```python
from build123d import *

# Parameters (mm, degrees)
SKETCH1_R           = 38.1
BOSS_EXTRUDE1_DEPTH = 4.826
SKETCH2_R           = 38.1
BOSS_EXTRUDE2_DEPTH = 3.302
BOSS_EXTRUDE2_DRAFT = -70
SKETCH3_R           = 47.172170439
BOSS_EXTRUDE3_DEPTH = 3.81
SKETCH4_R           = 46.472170439
CUT_EXTRUDE1_DEPTH  = 0.2
SKETCH6_R           = 34.772170439
SKETCH6_R_2         = 12.7
CUT_EXTRUDE2_DEPTH  = 2.7
SKETCH8_R           = 12.7
BOSS_EXTRUDE4_DEPTH = 50.8
SKETCH10_R          = 7.35
CUT_EXTRUDE5_DEPTH  = 3
SKETCH13_R          = 6.4
CUT_EXTRUDE9_DEPTH  = 92.577748235
SKETCH15_R          = 37.5
BOSS_EXTRUDE6_DEPTH = 8
CUT_EXTRUDE10_REACH = 99.233
SKETCH16_R          = 2
SKETCH16_R_2        = 5.35
SKETCH17_R          = 20.71
SKETCH17_R_2        = 19.21
CUT_EXTRUDE11_DEPTH = 3
SKETCH19_R          = 4.5
CUT_EXTRUDE12_DEPTH = 3.75


with BuildPart() as part:
    # Sketch1 → Boss-Extrude1 (new body)
    with BuildSketch(Plane(origin=(0, 0, 0), x_dir=(1, 0, 0), z_dir=(0, 1, 0))):
        with Locations(Location((0, 0, 0), (0, 0, 270))):
            Circle(SKETCH1_R)
    extrude(amount=BOSS_EXTRUDE1_DEPTH)


with BuildPart() as boss_extrude2_tool:
    # Sketch2 → Boss-Extrude2 (with draft: the straight prism first)
    with BuildSketch(Plane(origin=(0, 4.826, 0), x_dir=(1, 0, 0), z_dir=(0, 1, 0))):
        with Locations(Location((0, 0, 0), (0, 0, 270))):
            Circle(SKETCH2_R)
    extrude(amount=BOSS_EXTRUDE2_DEPTH)
    # Boss-Extrude2: the draft: its side faces are tilted about the plane it starts from
    boss_extrude2_sides = [boss_extrude2_tool.faces().sort_by_distance(p)[0] for p in [
        (0, 6.477, -38.1),
    ]]
    draft(boss_extrude2_sides, Plane(origin=(0, 4.826, 0), x_dir=(1, 0, 0), z_dir=(0, 1, 0)), BOSS_EXTRUDE2_DRAFT)


with BuildPart() as part_1:
    add(part.part)

    # Boss-Extrude2: add boss_extrude2_tool
    add(boss_extrude2_tool.part)

    # Sketch3 → Boss-Extrude3 (add)
    with BuildSketch(Plane(origin=(0, 8.128, 0), x_dir=(1, 0, 0), z_dir=(0, 1, 0))):
        with Locations(Location((0, 0, 0), (0, 0, 90))):
            Circle(SKETCH3_R)
    extrude(amount=BOSS_EXTRUDE3_DEPTH)

    # Sketch4 → Cut-Extrude1 (cut)
    with BuildSketch(Plane(origin=(0, 11.938, 0), x_dir=(1, 0, 0), z_dir=(0, 1, 0))):
        with Locations(Location((0, 0, 0), (0, 0, 270))):
            Circle(SKETCH4_R)
    extrude(amount=-CUT_EXTRUDE1_DEPTH, mode=Mode.SUBTRACT)

    # Sketch6 → Cut-Extrude2 (cut)
    with BuildSketch(Plane(origin=(0, 11.738, 0), x_dir=(1, 0, 0), z_dir=(0, 1, 0))):
        with Locations(Location((0, 0, 0), (0, 0, 270))):
            Circle(SKETCH6_R)
        with Locations(Location((0, 0, 0), (0, 0, 270))):
            Circle(SKETCH6_R_2, mode=Mode.SUBTRACT)
    extrude(amount=-CUT_EXTRUDE2_DEPTH, mode=Mode.SUBTRACT)

    # Sketch8 → Boss-Extrude4 (add)
    with BuildSketch(Plane.XZ):
        with Locations(Location((0, 0, 0), (0, 0, 90))):
            Circle(SKETCH8_R)
    extrude(amount=BOSS_EXTRUDE4_DEPTH)

    # Sketch10 → Cut-Extrude5 (cut)
    with BuildSketch(Plane(origin=(0, 11.738, 0), x_dir=(1, 0, 0), z_dir=(0, 1, 0))):
        with Locations(Location((0, 0, 0), (0, 0, 270))):
            Circle(SKETCH10_R)
    extrude(amount=-CUT_EXTRUDE5_DEPTH, mode=Mode.SUBTRACT)

    # Sketch13 → Cut-Extrude9 (cut, through all)
    with BuildSketch(Plane(origin=(0, -50.8, 0), x_dir=(-1, 0, 0), z_dir=(0, -1, 0))):
        with Locations(Location((0, 0, 0), (0, 0, 90))):
            Circle(SKETCH13_R)
    extrude(amount=-CUT_EXTRUDE9_DEPTH, mode=Mode.SUBTRACT)

    # Sketch15 → Boss-Extrude6 (add)
    with BuildSketch(Plane.XZ.offset(50.8)):
        with Locations(Location((0, 0, 0), (0, 0, 270))):
            Circle(SKETCH15_R)
    extrude(amount=BOSS_EXTRUDE6_DEPTH)

    # Sketch16 → Cut-Extrude10 (cut, up to next)
    with BuildSketch(Plane.XZ.offset(58.8), mode=Mode.PRIVATE) as cut_extrude10_sk1:
        with Locations(Location((0, 33.75, 0), (0, 0, 270))):
            Circle(SKETCH16_R)
    cut_extrude10_tool1 = extrude(cut_extrude10_sk1.sketch, amount=-CUT_EXTRUDE10_REACH, mode=Mode.PRIVATE) & part_1.part
    # Sketch16 → Cut-Extrude10 (cut, up to next)
    with BuildSketch(Plane.XZ.offset(58.8), mode=Mode.PRIVATE) as cut_extrude10_sk2:
        with Locations(Location((23.864853865, 23.864853865, 0), (0, 0, 270))):
            Circle(SKETCH16_R)
    cut_extrude10_tool2 = extrude(cut_extrude10_sk2.sketch, amount=-CUT_EXTRUDE10_REACH, mode=Mode.PRIVATE) & part_1.part
    # Sketch16 → Cut-Extrude10 (cut, up to next)
    with BuildSketch(Plane.XZ.offset(58.8), mode=Mode.PRIVATE) as cut_extrude10_sk3:
        with Locations(Location((33.75, 0, 0), (0, 0, 270))):
            Circle(SKETCH16_R)
    cut_extrude10_tool3 = extrude(cut_extrude10_sk3.sketch, amount=-CUT_EXTRUDE10_REACH, mode=Mode.PRIVATE) & part_1.part
    # Sketch16 → Cut-Extrude10 (cut, up to next)
    with BuildSketch(Plane.XZ.offset(58.8), mode=Mode.PRIVATE) as cut_extrude10_sk4:
        with Locations(Location((23.864853865, -23.864853865, 0), (0, 0, 270))):
            Circle(SKETCH16_R)
    cut_extrude10_tool4 = extrude(cut_extrude10_sk4.sketch, amount=-CUT_EXTRUDE10_REACH, mode=Mode.PRIVATE) & part_1.part
    # Sketch16 → Cut-Extrude10 (cut, up to next)
    with BuildSketch(Plane.XZ.offset(58.8), mode=Mode.PRIVATE) as cut_extrude10_sk5:
        with Locations(Location((0, -33.75, 0), (0, 0, 270))):
            Circle(SKETCH16_R)
    cut_extrude10_tool5 = extrude(cut_extrude10_sk5.sketch, amount=-CUT_EXTRUDE10_REACH, mode=Mode.PRIVATE) & part_1.part
    # Sketch16 → Cut-Extrude10 (cut, up to next)
    with BuildSketch(Plane.XZ.offset(58.8), mode=Mode.PRIVATE) as cut_extrude10_sk6:
        with Locations(Location((-23.864853865, -23.864853865, 0), (0, 0, 270))):
            Circle(SKETCH16_R)
    cut_extrude10_tool6 = extrude(cut_extrude10_sk6.sketch, amount=-CUT_EXTRUDE10_REACH, mode=Mode.PRIVATE) & part_1.part
    # Sketch16 → Cut-Extrude10 (cut, up to next)
    with BuildSketch(Plane.XZ.offset(58.8), mode=Mode.PRIVATE) as cut_extrude10_sk7:
        with Locations(Location((-33.75, 0, 0), (0, 0, 270))):
            Circle(SKETCH16_R)
    cut_extrude10_tool7 = extrude(cut_extrude10_sk7.sketch, amount=-CUT_EXTRUDE10_REACH, mode=Mode.PRIVATE) & part_1.part
    # Sketch16 → Cut-Extrude10 (cut, up to next)
    with BuildSketch(Plane.XZ.offset(58.8), mode=Mode.PRIVATE) as cut_extrude10_sk8:
        with Locations(Location((-23.864853865, 23.864853865, 0), (0, 0, 270))):
            Circle(SKETCH16_R)
    cut_extrude10_tool8 = extrude(cut_extrude10_sk8.sketch, amount=-CUT_EXTRUDE10_REACH, mode=Mode.PRIVATE) & part_1.part
    # Sketch16 → Cut-Extrude10 (cut, up to next)
    with BuildSketch(Plane.XZ.offset(58.8), mode=Mode.PRIVATE) as cut_extrude10_sk9:
        with Locations(Location((0, 0, 0), (0, 0, 270))):
            Circle(SKETCH16_R_2)
    cut_extrude10_tool9 = extrude(cut_extrude10_sk9.sketch, amount=-CUT_EXTRUDE10_REACH, mode=Mode.PRIVATE) & part_1.part
    add(cut_extrude10_tool1.solids().sort_by_distance((0, -58.8, 33.75))[0], mode=Mode.SUBTRACT)
    add(cut_extrude10_tool2.solids().sort_by_distance((23.864854, -58.8, 23.864854))[0], mode=Mode.SUBTRACT)
    add(cut_extrude10_tool3.solids().sort_by_distance((33.75, -58.8, 0))[0], mode=Mode.SUBTRACT)
    add(cut_extrude10_tool4.solids().sort_by_distance((23.864854, -58.8, -23.864854))[0], mode=Mode.SUBTRACT)
    add(cut_extrude10_tool5.solids().sort_by_distance((0, -58.8, -33.75))[0], mode=Mode.SUBTRACT)
    add(cut_extrude10_tool6.solids().sort_by_distance((-23.864854, -58.8, -23.864854))[0], mode=Mode.SUBTRACT)
    add(cut_extrude10_tool7.solids().sort_by_distance((-33.75, -58.8, 0))[0], mode=Mode.SUBTRACT)
    add(cut_extrude10_tool8.solids().sort_by_distance((-23.864854, -58.8, 23.864854))[0], mode=Mode.SUBTRACT)
    add(cut_extrude10_tool9.solids().sort_by_distance((0, -58.8, 0))[0], mode=Mode.SUBTRACT)

    # Sketch17 → Cut-Extrude11 (cut)
    with BuildSketch(Plane.XZ.offset(58.8)):
        with Locations(Location((0, 0, 0), (0, 0, 270))):
            Circle(SKETCH17_R)
        with Locations(Location((0, 0, 0), (0, 0, 270))):
            Circle(SKETCH17_R_2, mode=Mode.SUBTRACT)
    extrude(amount=-CUT_EXTRUDE11_DEPTH, mode=Mode.SUBTRACT)

    # Sketch19 → Cut-Extrude12 (cut)
    with BuildSketch(Plane(origin=(0, -50.8, 0), x_dir=(1, 0, 0), z_dir=(0, 1, 0))):
        with Locations((23.864853865, 23.864853865)):
            Circle(SKETCH19_R)
        with Locations((0, 33.75)):
            Circle(SKETCH19_R)
        with Locations((33.75, 0)):
            Circle(SKETCH19_R)
        with Locations((23.864853865, -23.864853865)):
            Circle(SKETCH19_R)
        with Locations((0, -33.75)):
            Circle(SKETCH19_R)
        with Locations((-23.864853865, -23.864853865)):
            Circle(SKETCH19_R)
        with Locations((-33.75, 0)):
            Circle(SKETCH19_R)
        with Locations((-23.864853865, 23.864853865)):
            Circle(SKETCH19_R)
    extrude(amount=-CUT_EXTRUDE12_DEPTH, mode=Mode.SUBTRACT)


solid = part_1.part
```
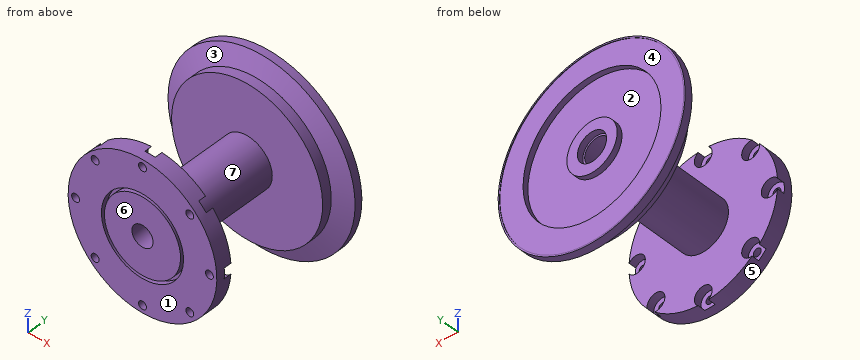
Geometry check sheet. Reference: the model listing, model coordinates, mm. Face numbers are marked on the shaded views. A direction names the side the tool comes from. Coordinates: 2 decimals unless noted, no trailing zeros. Order: outer loops, then holes, each group sorted by start corner. A loop starts at its lowest first (then second) coordinate and runs counter-clockwise, first axis right, second up. Notation, with made-up numbers: (32, -24.5) - (67, -24.5) arc R32 cw to (67, 9.5) - close; hole circle Ø1 at (-2.5, 4.25). An arc over 180 degrees is marked (long way). Answer as a JSON object with one key per item and string values. Group by question number.
Item 1: Tool access check on the marked faces 4, 5, 6 and 7. Record the directions out of +Z, -Z, +X, -X, +Y, -Y that give a thin tool (end or side, any length) a straight path to the whole face; none if there is none.
Item 2: Sectioned sample at B-B, the plane y = 2. Record the cut outline in (x, z), and give its area (3 significant figures).
Item 3: Depth check by flat-ended pin: pin 1 Ø2.5 at (x, z) = (23.86, -23.86) entering from -Y; pin 2 Ø8 at (x, z) = (23.86, 23.86) entering from -Y; pin 3 Ø5 at (x, z) = (3.5, 8) entering from +Y; pin 4 Ø10 at (x, y) = (-6, -31) entering from -Z. Enter the tip coordinate at first touch or a pass-through.
Item 4: Scan lines: probe 1 along X at (y, z) = (-25.5, 0); probe 2 along X at (y, z) = (-55, 0); probe 3 along Y at (x, z) = (15.5, 4). Record each from-to range of solid material in increasing order.
Item 5: Draft check along Z on the marked faces 1, 2 and 3. Enter one of: +Z half, -Z half, draft (parallel to the pull), parting line (faces both ways), or undercut.
Item 6: Sectioned sample at A-A, the plane x = 0. Give the number of separate pieces and of enclosed holes in the cut face, and give its area (3 significant figures).
Resolved:
{
 "1": {"face 4": "+Y", "face 5": "-Y", "face 6": "+Z, -Z, +X, -X, -Y", "face 7": "none"},
 "2": {"outline": "circle Ø76.2 at (0, 0); hole circle Ø12.8 at (0, 0)", "area": "4,430 mm^2"},
 "3": {"pin 1": "y = 0", "pin 2": "y = -58.8", "pin 3": "y = 11.74", "pin 4": "z = -12.66"},
 "4": {"probe 1": "-12.7 to -6.4, 6.4 to 12.7", "probe 2": "-37.5 to -35.75, -31.75 to -5.35, 5.35 to 31.75, 35.75 to 37.5", "probe 3": "-58.8 to -50.8, 0 to 9.04"},
 "5": {"face 1": "draft", "face 2": "undercut", "face 3": "parting line"},
 "6": {"separate pieces": "4", "enclosed holes": "0", "area": "1,760 mm^2"}
}
